```python
from build123d import *

# Parameters (mm, degrees)
SKETCH1_W           = 90
SKETCH1_H           = 55
SKETCH1_W_2         = 6.35
SKETCH1_H_2         = 30
SKETCH1_H_3         = 50
BOSS_EXTRUDE1_DEPTH = 2
SKETCH2_R           = 2.5
BOSS_EXTRUDE2_DEPTH = 10
SKETCH3_R           = 1.25
BOSS_EXTRUDE3_DEPTH = 3
FILLET1_R           = 2
FILLET2_R           = 1


with BuildPart() as part:
    # Sketch1 → Boss-Extrude1 (new body)
    with BuildSketch(Plane(origin=(0, 0, 0), x_dir=(1, 0, 0), z_dir=(0, 1, 0))):
        with Locations((45, 27.5)):
            Rectangle(SKETCH1_W, SKETCH1_H)
        with Locations((83.825, 17.5)):
            Rectangle(SKETCH1_W_2, SKETCH1_H_2, mode=Mode.SUBTRACT)
        with Locations((6.175, 27.5)):
            Rectangle(SKETCH1_W_2, SKETCH1_H_3, mode=Mode.SUBTRACT)
    extrude(amount=BOSS_EXTRUDE1_DEPTH)

    # Sketch2 → Boss-Extrude2 (add)
    with BuildSketch(Plane(origin=(0, 2, 0), x_dir=(1, 0, 0), z_dir=(0, 1, 0))):
        with Locations(Location((34, 51.5, 0), (0, 0, 90))):
            Circle(SKETCH2_R)
        with Locations(Location((34, 3.5, 0), (0, 0, 90))):
            Circle(SKETCH2_R)
        with Locations(Location((86, 37.5, 0), (0, 0, 90))):
            Circle(SKETCH2_R)
    extrude(amount=BOSS_EXTRUDE2_DEPTH)

    # Sketch3 → Boss-Extrude3 (add)
    with BuildSketch(Plane(origin=(0, 12, 0), x_dir=(1, 0, 0), z_dir=(0, 1, 0))):
        with Locations(Location((34, 51.5, 0), (0, 0, 270))):
            Circle(SKETCH3_R)
        with Locations(Location((34, 3.5, 0), (0, 0, 270))):
            Circle(SKETCH3_R)
        with Locations(Location((86, 37.5, 0), (0, 0, 270))):
            Circle(SKETCH3_R)
    extrude(amount=BOSS_EXTRUDE3_DEPTH)

    # Fillet1
    fillet1_edges = [part.edges().sort_by_distance(p)[0] for p in [
        (80.65, 1, -32.5),
        (80.65, 1, -2.5),
        (87, 1, -2.5),
        (87, 1, -32.5),
        (3, 1, -52.5),
        (3, 1, -2.5),
        (9.35, 1, -2.5),
        (9.35, 1, -52.5),
        (0, 1, -55),
        (90, 1, -55),
        (90, 1, 0),
        (0, 1, 0),
    ]]
    fillet(fillet1_edges, radius=FILLET1_R)

    # Fillet2
    fillet2_edges = [part.edges().sort_by_distance(p)[0] for p in [
        (86, 2, -35),
        (34, 2, -1),
        (34, 2, -49),
    ]]
    fillet(fillet2_edges, radius=FILLET2_R - 0.0001)  # a hair under: the kernel refuses the full size


solid = part.part
```
Work out the finished part from the listing and answer in its coordinate system (mm). A direction names the side the tool comes from. Give positions to 0.01 mm unless a question says otherwise; leave off trailing zeros. Write each loop counter-clockwise with the first axis right and the second up, starting at its lowest first coordinate (ties: lowest second). Pieces come first, ordered by that corner, then holes.
(1) Which of the six approach directions +Z, -Z, +X, -X, +Y, -Y give full straight-line access (tool end or side, diameter ignored) to faces 1 (the cylindrical face through (8.75, 1.01, -3.07)), 2 (the cylindrical face through (32.891, 13.479, -2.923)), 3 (the flat face through (90, 1, -27))?
Final values:
face 1: +Y, -Y
face 2: +Y
face 3: +Z, -Z, +X, +Y, -Y
(2) The part is cut by section A-A on z = -37.5. Write down the section's boundary in (x, y), plus the area to 3 significant figures.
Final values:
outline: (0, 0) - (3, 0) - (3, 2) - (0, 2) - close; (9.35, 0) - (90, 0) - (90, 2) - (89.5, 2) arc R1 cw to (88.5, 3) - (88.5, 12) - (87.25, 12) - (87.25, 15) - (84.75, 15) - (84.75, 12) - (83.5, 12) - (83.5, 3) arc R1 cw to (82.5, 2) - (9.35, 2) - close
area: 225 mm2
(3) The part is cut by section C-C on z = -16.5. Write down the section's boundary in (x, y).
Final values:
outline: (0, 0) - (3, 0) - (3, 2) - (0, 2) - close; (9.35, 0) - (80.65, 0) - (80.65, 2) - (9.35, 2) - close; (87, 0) - (90, 0) - (90, 2) - (87, 2) - close
(4) The part is cut by section D-D on x = 86. Write down the section's boundary in (y, z).
Final values:
outline: (0, -55) - (2, -55) - (2, -41) arc R1 cw to (3, -40) - (12, -40) - (12, -38.75) - (15, -38.75) - (15, -36.25) - (12, -36.25) - (12, -35) - (3, -35) arc R1 cw to (2, -34) - (2, -32.23) - (0, -32.23) - close; (0, -2.77) - (2, -2.77) - (2, 0) - (0, 0) - close
(5) Flat-ended cylindrical pins translate along their axes: pin 1 Ø10 at (x, z) = (79, -32) entering from +Y; pin 2 Ø4 at (x, z) = (37.5, -5.5) entering from +Y. Find the tip coordinate at first contact, or state that the pin passes through.
Final values:
pin 1: stops at y = 2
pin 2: stops at y = 12
(6) The mould has two halves that part along Z. Classify faces 4 (the cylindrical face through (3.6, 1.01, -51.93)), 5 (the flat face through (34, 15, -52)), 6 (the cylindrical face through (0.57, 1.01, -54.4)): pulls with the +Z half, pulls with the -Z half, needs draft (parallel to the pull), parting line crosses it, or undercut.
Final values:
face 4: undercut
face 5: needs draft
face 6: pulls with the -Z half
(7) Straight lines are drawn through the part: line 1 (Y direction, x = 49, z = -49); line 2 (X direction, y = 1.5, z = -41.5); line 3 (X direction, y = 6.5, z = -36.5). For each, find the intervals that lie inside material, in ascending order.
Final values:
line 1: y = 0 to 2
line 2: x = 0 to 3, 9.35 to 90
line 3: x = 83.71 to 88.29
(8) The part is cut by section B-B on y = 14. Write down the section's boundary in (x, z).
Final values:
outline: circle Ø2.5 at (34, -51.5); circle Ø2.5 at (34, -3.5); circle Ø2.5 at (86, -37.5)
